Model file for the job. Use its own axes, mm. Face numbers are marked on the shaded views. A direction names the side the tool comes from. Round coordinates to 2 decimals unless told otherwise and drop trailing zeros. Loops run counter-clockwise (first coordinate to the right, second up) from the corner with the lowest first, then second, coordinate; pieces in that order, holes last. Notation, with made-up numbers: (87.25, 2) - (122.25, 2) arc R22 ccw to (122.25, 33) - close; hole circle Ø1 at (28, 12). An arc over 180 degrees is marked (long way). Answer as a JSON object with one key per item and string values.
from build123d import *

# Parameters (mm, degrees)
SALIENTE_EXTRUIR1_DEPTH      = 2.5
SALIENTE_EXTRUIR1_DEPTH_BACK = 2.5
CROQUIS1_W                   = 3
CROQUIS1_H                   = 50
SALIENTE_EXTRUIR2_DEPTH      = 5
SALIENTE_EXTRUIR2_DEPTH_BACK = 5
CROQUIS1_3_R                 = 1.5


with BuildPart() as part:
    # Croquis1 → Saliente-Extruir1 (new, two sides: drawn at the far end of the back side and taken through both)
    with BuildSketch(Plane.XY.offset(-SALIENTE_EXTRUIR1_DEPTH_BACK)):
        Rectangle(CROQUIS1_W, CROQUIS1_H)
    extrude(amount=SALIENTE_EXTRUIR1_DEPTH + SALIENTE_EXTRUIR1_DEPTH_BACK)

    # Croquis1<3> → Saliente-Extruir2 (add, two sides: drawn at the far end of the back side and taken through both)
    with BuildSketch(Plane.XY.offset(-SALIENTE_EXTRUIR2_DEPTH_BACK)):
        with Locations((0, 25)):
            Circle(CROQUIS1_3_R)
        with Locations((0, -25)):
            Circle(CROQUIS1_3_R)
        Circle(CROQUIS1_3_R)
    extrude(amount=SALIENTE_EXTRUIR2_DEPTH + SALIENTE_EXTRUIR2_DEPTH_BACK)


solid = part.part
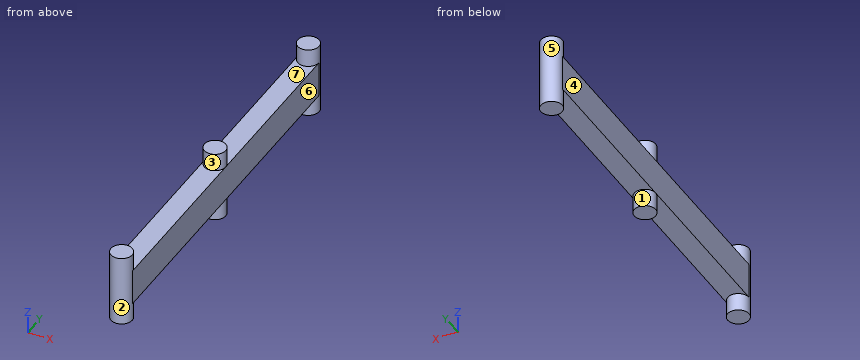
1) Probe probe 1 along Y at (x, z) = (0.8, 3.25); probe 2 along Y at (x, z) = (1.2, 2.75); probe 3 along Z at (x, y) = (-0.95, 9). List the from-to ranges inside material, lowest first.
Values follow:
{"probe 1": "-26.27 to -23.73, -1.27 to 1.27, 23.73 to 26.27", "probe 2": "-25.9 to -24.1, -0.9 to 0.9, 24.1 to 25.9", "probe 3": "-2.5 to 2.5"}
2) Slice it at A-A on x = 0. List the corners of the cut face in (y, z).
Values follow:
{"outline": "(-26.5, -5) - (-23.5, -5) - (-23.5, -2.5) - (-1.5, -2.5) - (-1.5, -5) - (1.5, -5) - (1.5, -2.5) - (23.5, -2.5) - (23.5, -5) - (26.5, -5) - (26.5, 5) - (23.5, 5) - (23.5, 2.5) - (1.5, 2.5) - (1.5, 5) - (-1.5, 5) - (-1.5, 2.5) - (-23.5, 2.5) - (-23.5, 5) - (-26.5, 5) - close"}
3) Drop a flat-ended pin along its axis: P1, Ø1.5, axis at x = 0, y = -9.5, coming from the +Z side. Give the stop position or say it passes through.
Values follow:
{"P1": "z = 2.5"}
4) Two-plate mould, pull along Y, no slides. Class the marked faces 5, 6 and 7: pulls with the +Y half, pulls with the -Y half, needs draft (parallel to the pull), parting line crosses it, or undercut.
Values follow:
{"face 5": "undercut", "face 6": "needs draft", "face 7": "undercut"}
5) Slice it at C-C on y = -16. List the corners of the cut face in (x, z), then the cut area to 3 significant figures.
Values follow:
{"outline": "(-1.5, -2.5) - (1.5, -2.5) - (1.5, 2.5) - (-1.5, 2.5) - close", "area": "15.0 mm²"}
6) Slice it at B-B on z = -3.25. List the corners of the cut face in (x, y), then the cut area to 3 significant figures.
Values follow:
{"outline": "circle Ø3 at (0, -25); circle Ø3 at (0, 0); circle Ø3 at (0, 25)", "area": "21.2 mm²"}
7) Tool access for the marked faces 1, 2, 3 and 4: list every direction of +Z, -Z, +X, -X, +Y, -Y with a clear straight run to the whole face (end or side of a thin tool).
Values follow:
{"face 1": "-Z", "face 2": "none", "face 3": "+Z", "face 4": "+Z, -Z, -X, +Y, -Y"}
